Check sheet for the drawn part. Datum: minimum x, y, z corner. Units: mm. A direction names the side the tool comes from. Round coordinates to 2 decimals unless told otherwise and drop trailing zeros. Write each loop counter-clockwise with the first axis right and the second up, starting at its lowest first coordinate (ties: lowest second). Pieces come first, ordered by that corner, then holes. Notation, with made-up numbers: (0, 48) - (17, 48) arc R25 cw to (17, 67) - close; hole circle Ø5 at (25.5, 51.25). An arc over 180 degrees is marked (long way). Answer as a JSON object with one key per item and string values. Group by question number.
Item 1: Set-up check for the marked faces 1 and 2: record each of +Z, -Z, +X, -X, +Y, -Y from which the full face is reachable in a straight line by a thin tool's end or side.
Item 2: Thickness scan on line 1 (Z direction, x = 1.75, y = 1.25); line 2 (Y direction, x = 6.75, z = 7.5); line 3 (X direction, y = 5.75, z = 8). Record the ranges inside material, lowest first.
Item 3: Sectioned sample at C-C on z = 9.5. Record the boundary of the cut face in (x, y), plus the area to 3 significant figures.
Item 4: Sectioned sample at B-B on y = 6.25. Record the boundary of the cut face in (x, z), plus the area to 3 significant figures.
Item 5: Sectioned sample at D-D on y = 10.25. Record the boundary of the cut face in (x, z).
Item 6: Sectioned sample at A-A on x = 6.7. Record the boundary of the cut face in (y, z).
Item 7: Gauge pin test, flat end, axial feed: P1, Ø6, axis at x = 5, z = 10, coming from the -Y side. Record the tip position at first contact, or that the pin passes through.
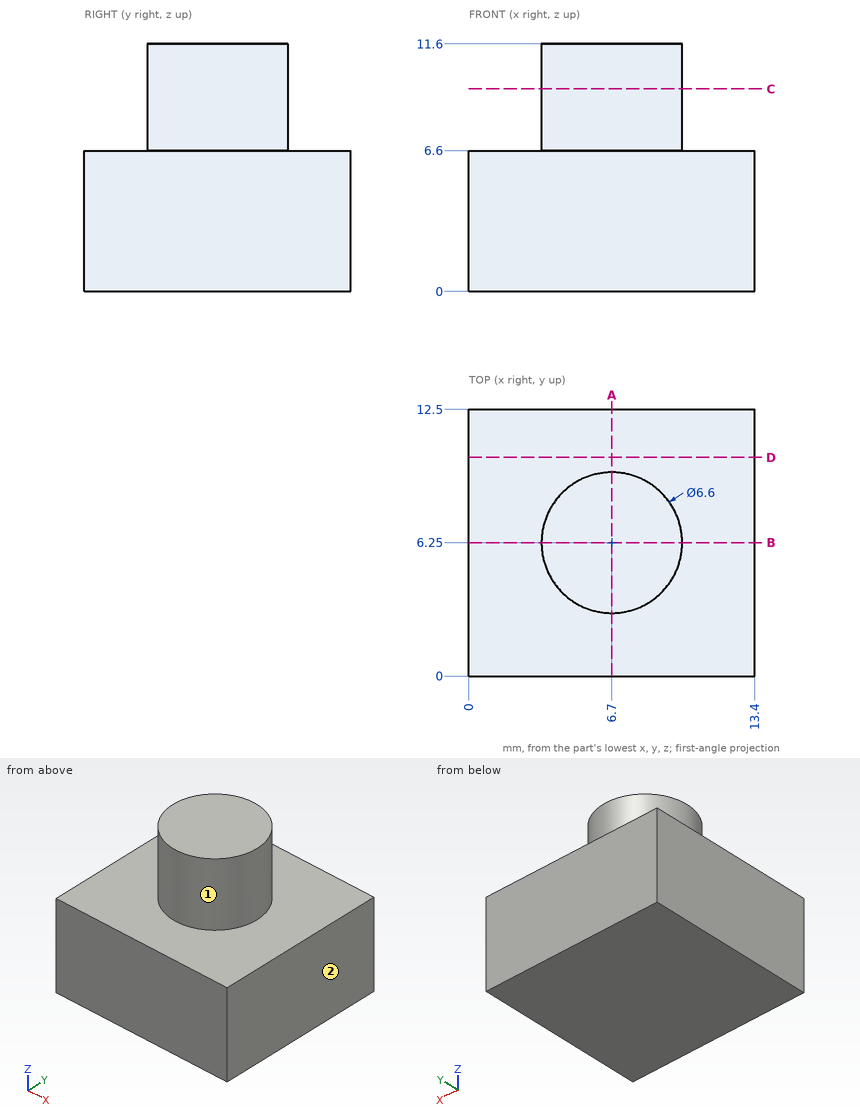
Completed:
{
 "1": {"face 1": "+Z", "face 2": "+Z, -Z, +X, +Y, -Y"},
 "2": {"line 1": "0 to 6.6", "line 2": "2.95 to 9.55", "line 3": "3.44 to 9.96"},
 "3": {"outline": "circle Ø6.6 at (6.7, 6.25)", "area": "34.2 mm²"},
 "4": {"outline": "(0, 0) - (13.4, 0) - (13.4, 6.6) - (10, 6.6) - (10, 11.6) - (3.4, 11.6) - (3.4, 6.6) - (0, 6.6) - close", "area": "121 mm²"},
 "5": {"outline": "(0, 0) - (13.4, 0) - (13.4, 6.6) - (0, 6.6) - close"},
 "6": {"outline": "(0, 0) - (12.5, 0) - (12.5, 6.6) - (9.55, 6.6) - (9.55, 11.6) - (2.95, 11.6) - (2.95, 6.6) - (0, 6.6) - close"},
 "7": {"P1": "y = 2.95"}
}
